The listing builds one solid part. Answer for the finished solid, in the listing's coordinates (mm). A direction names the side the tool comes from. Give positions to 0.01 mm unless a question says otherwise; leave off trailing zeros. Order: outer loops, then holes, each group sorted by start corner. A loop starts at its lowest first (then second) coordinate and runs counter-clockwise, first axis right, second up. Notation, with made-up numbers: (-2, 64.25) -> (40, 64.25) arc R25 ccw to (40, 103.25) -> close; hole circle Ø11 at (-10.75, 29). An arc over 180 degrees is marked (long way). Write item = value, one per line. Start each with the question number.
```python
from build123d import *

# Parameters (mm, degrees)
SKETCH1_W           = 20
SKETCH1_H           = 20
SKETCH1_R           = 3.2
BOSS_EXTRUDE1_DEPTH = 4
SKETCH2_W           = 20
SKETCH2_H           = 4
BOSS_EXTRUDE2_DEPTH = 15
CUT_EXTRUDE1_DEPTH  = 15
BOSS_EXTRUDE3_DEPTH = 4
SKETCH5_R           = 1.7
CUT_EXTRUDE2_DEPTH  = 4
FILLET1_R           = 3
FILLET2_R           = 3


with BuildPart() as part:
    # Sketch1 → Boss-Extrude1 (new body)
    with BuildSketch(Plane.XY):
        Rectangle(SKETCH1_W, SKETCH1_H)
        Circle(SKETCH1_R, mode=Mode.SUBTRACT)
    extrude(amount=BOSS_EXTRUDE1_DEPTH)

    # Sketch2 → Boss-Extrude2 (add)
    with BuildSketch(Plane.XY.offset(4)):
        with Locations((0, -8)):
            Rectangle(SKETCH2_W, SKETCH2_H)
    extrude(amount=BOSS_EXTRUDE2_DEPTH)

    # Sketch3 → Cut-Extrude1 (cut)
    with BuildSketch(Plane(origin=(0, -6, 0), x_dir=(1, 0, 0), z_dir=(0, 1, 0))):
        Polygon((-10, -19), (-10, -4), (6, -19), align=None)
    extrude(amount=-CUT_EXTRUDE1_DEPTH, mode=Mode.SUBTRACT)

    # Sketch4 → Boss-Extrude3 (add)
    with BuildSketch(Plane(origin=(10, 0, 0), x_dir=(0, 0, -1), z_dir=(1, 0, 0))):
        Polygon((0, -10), (-15, -26), (-19, -26), (-19, -10), align=None)
    extrude(amount=-BOSS_EXTRUDE3_DEPTH)

    # Sketch5 → Cut-Extrude2 (cut)
    with BuildSketch(Plane(origin=(10, 0, 0), x_dir=(0, 0, -1), z_dir=(1, 0, 0))):
        with Locations((-16.059117511, -22.587455859)):
            Circle(SKETCH5_R)
    extrude(amount=-CUT_EXTRUDE2_DEPTH, mode=Mode.SUBTRACT)

    # Fillet1
    # the kernel refuses this fillet: 3 mm, written as the material it takes off along each edge
    with BuildSketch(Plane(origin=(13.249240093, -26, 15), x_dir=(0, 0.7295372041400854, -0.6839411288813294), z_dir=(-1, 0, 0))) as fillet1_piece_1:
        with BuildLine():
            CenterArc((FILLET1_R * 0.433232012466, -FILLET1_R), FILLET1_R, 90, 46.847610266)
            Line((-FILLET1_R * 0.296305191674, -FILLET1_R * 0.316058871119), (0, 0))
            Line((0, 0), (FILLET1_R * 0.433232012466, 0))
        make_face()
    extrude(amount=10.498480187, mode=Mode.SUBTRACT)
    with BuildSketch(Plane(origin=(17.5, -26, 19), x_dir=(0, 0, -1), z_dir=(-1, 0, 0))) as fillet1_piece_2:
        with BuildLine():
            CenterArc((FILLET1_R, -FILLET1_R), FILLET1_R, 90, 90)
            Line((0, -FILLET1_R), (0, 0))
            Line((0, 0), (FILLET1_R, 0))
        make_face()
    extrude(amount=19, mode=Mode.SUBTRACT)

    # Fillet2
    fillet2_edges = [part.edges().sort_by_distance(p)[0] for p in [
        (8, -6, 19),
        (-10, -10, 2),
        (-10, 10, 2),
        (10, 10, 2),
    ]]
    fillet(fillet2_edges, radius=FILLET2_R)


solid = part.part
```
Item 1: A cutting plane is placed at B-B, the plane x = 2. Write down the section's boundary in (y, z), plus the area to 3 significant figures.
Item 2: A cutting plane is placed at C-C, the plane z = 6.25. Write down the section's boundary in (x, y), plus the area to 3 significant figures.
Item 3: Consider L1, parallel to Y at x = 0, z = 1.15; L2, parallel to Z at x = -8.75, y = -1; L3, parallel to Y at x = -0.25, z = 7. Determine where each line is inside the solid, lowest interval first. Write a range as from..to.
Item 4: The mould has two halves that part along Y. Classify faces 1 (the cylindrical face through (-2.539, -1.947, 1.972)), 2 (the cylindrical face through (-9.14, 9.1, 2.03)), 3 (the flat face through (-2.4, 2.4, 0)), 4 (the flat face through (8.028, -17.421, 6.957)): +Y half, -Y half, draft (parallel to the pull), parting line (faces both ways), or undercut.
Item 5: Which of the six approach directions +Z, -Z, +X, -X, +Y, -Y give full straight-line access (tool end or side, diameter ignored) to faces 5 (the flat face through (-2.112, -7.972, 11.395)), 6 (the flat face through (1, -10, 7)), 7 (the flat face through (0, 4, 4))?
Item 6: A cutting plane is placed at D-D, the plane x = 0. Write down the section's boundary in (y, z) (3 decimals), plus the area to 3 significant figures.
Item 7: A cutting plane is placed at A-A, the plane y = 0. Write down the section's boundary in (x, z), plus the area to 3 significant figures.
Item 8: Flat-ended cylindrical pins translate along their axes: pin 1 (3.5 mm diameter, centred on x = -2, z = 11, fed in from +Y); pin 2 (5 mm diameter, centred on x = 2, y = 0, fed in from +Z); pin 3 (4 mm diameter, centred on y = -5.5, z = 8.5, fed in from -X); pin 4 (1.5 mm diameter, centred on x = -7.5, z = 10, fed in from -Y). Find the tip coordinate at first contact, or state that the pin passes through.
Check values:
q1.outline = (-10, 0) -> (-2.5, 0) -> (-2.5, 4) -> (-6, 4) -> (-6, 15.25) -> (-10, 15.25) -> close; (2.5, 0) -> (10, 0) -> (10, 4) -> (2.5, 4) -> close
q1.area = 105 mm^2
q2.outline = (-7.6, -9.94) arc R3 ccw to (-7, -10) -> (6, -10) -> (6, -16.67) -> (10, -16.67) -> (10, -6) -> (-7.6, -6) -> close
q2.area = 97.1 mm^2
q3.L1 = -10..-3.2, 3.2..10
q3.L2 = 0..4
q3.L3 = -10..-6
q4.face_1 = undercut
q4.face_2 = +Y half
q4.face_3 = draft
q4.face_4 = -Y half
q5.face_5 = +Z, -X, +Y, -Y
q5.face_6 = +Z, -Z, -X, -Y
q5.face_7 = +Z, +X, -X, +Y
q6.outline = (-10, 0) -> (-3.2, 0) -> (-3.2, 4) -> (-6, 4) -> (-6, 13.375) -> (-10, 13.375) -> close; (3.2, 0) -> (10, 0) -> (10, 4) -> (3.2, 4) -> close
q6.area = 91.9 mm^2
q7.outline = (-10, 0) -> (-3.2, 0) -> (-3.2, 4) -> (-10, 4) -> close; (3.2, 0) -> (10, 0) -> (10, 4) -> (3.2, 4) -> close
q7.area = 54.4 mm^2
q8.pin_1 = -6
q8.pin_2 = 4
q8.pin_3 = -7.27
q8.pin_4 = through
